```python
from build123d import *

# Parameters (mm, degrees)
SKETCH1_W           = 50
SKETCH1_H           = 80
BOSS_EXTRUDE1_DEPTH = 9.5
CUT_EXTRUDE1_DEPTH  = 10.5
CUT_EXTRUDE2_DEPTH  = 4


with BuildPart() as part:
    # Sketch1 → Boss-Extrude1 (new body)
    with BuildSketch(Plane(origin=(0, 0, 0), x_dir=(1, 0, 0), z_dir=(0, 1, 0))):
        Rectangle(SKETCH1_W, SKETCH1_H)
    extrude(amount=BOSS_EXTRUDE1_DEPTH)

    # Sketch2 → Cut-Extrude1 (cut, through all)
    with BuildSketch(Plane(origin=(0, 9.5, 0), x_dir=(1, 0, 0), z_dir=(0, 1, 0))):
        with BuildLine():
            Line((-13.9, 35), (-13.9, 31))
            ThreePointArc((-13.9, 31), (-15.5, 29.4), (-17.1, 31))
            Line((-17.1, 31), (-17.1, 35))
            ThreePointArc((-17.1, 35), (-15.5, 36.6), (-13.9, 35))
        make_face()
        with BuildLine():
            Line((13.9, 35), (13.9, 31))
            ThreePointArc((13.9, 31), (15.5, 29.4), (17.1, 31))
            Line((17.1, 31), (17.1, 35))
            ThreePointArc((17.1, 35), (15.5, 36.6), (13.9, 35))
        make_face()
        with BuildLine():
            Line((-13.9, 4), (-13.9, 0))
            ThreePointArc((-13.9, 0), (-15.5, -1.6), (-17.1, 0))
            Line((-17.1, 0), (-17.1, 4))
            ThreePointArc((-17.1, 4), (-15.5, 5.6), (-13.9, 4))
        make_face()
        with BuildLine():
            Line((13.9, 4), (13.9, 0))
            ThreePointArc((13.9, 0), (15.5, -1.6), (17.1, 0))
            Line((17.1, 0), (17.1, 4))
            ThreePointArc((17.1, 4), (15.5, 5.6), (13.9, 4))
        make_face()
        with BuildLine():
            Line((8.5, 19.5), (8.5, 15.5))
            ThreePointArc((8.5, 15.5), (0, 7), (-8.5, 15.5))
            Line((-8.5, 15.5), (-8.5, 19.5))
            ThreePointArc((-8.5, 19.5), (0, 28), (8.5, 19.5))
        make_face()
    extrude(amount=-CUT_EXTRUDE1_DEPTH, mode=Mode.SUBTRACT)

    # Sketch3 → Cut-Extrude2 (cut)
    with BuildSketch(Plane(origin=(0, 9.5, 0), x_dir=(1, 0, 0), z_dir=(0, 1, 0))):
        with BuildLine():
            Line((12, 19.5), (12, 15.358826141))
            ThreePointArc((12, 15.358826141), (0, 3.358826141), (-12, 15.358826141))
            Line((-12, 15.358826141), (-12, 19.5))
            ThreePointArc((-12, 19.5), (0, 31.5), (12, 19.5))
        make_face()
    extrude(amount=-CUT_EXTRUDE2_DEPTH, mode=Mode.SUBTRACT)


solid = part.part
```
Work out the finished part from the listing and answer in its coordinate system (mm). A direction names the side the tool comes from. Coordinates: 2 decimals unless noted, no trailing zeros. Loops run counter-clockwise (first coordinate to the right, second up) from the corner with the lowest first, then second, coordinate; pieces in that order, holes last.
1) Section B-B (y = 2.75) is taken. Give the vertices of the cut face in (x, z).
Results:
outline: (-25, -40) - (25, -40) - (25, 40) - (-25, 40) - close; hole (-17.1, -35) arc R1.6 ccw to (-13.9, -35) - (-13.9, -31) arc R1.6 ccw to (-17.1, -31) - close; hole (-17.1, -4) arc R1.6 ccw to (-13.9, -4) - (-13.9, 0) arc R1.6 ccw to (-17.1, 0) - close; hole (-8.5, -19.5) arc R8.5 ccw to (8.5, -19.5) - (8.5, -15.5) arc R8.5 ccw to (-8.5, -15.5) - close; hole (13.9, -35) arc R1.6 ccw to (17.1, -35) - (17.1, -31) arc R1.6 ccw to (13.9, -31) - close; hole (13.9, -4) arc R1.6 ccw to (17.1, -4) - (17.1, 0) arc R1.6 ccw to (13.9, 0) - close
2) Section A-A (x = 15.5) is taken. Give the vertices of the cut face in (y, z).
Results:
outline: (0, -40) - (9.5, -40) - (9.5, -36.6) - (0, -36.6) - close; (0, -29.4) - (9.5, -29.4) - (9.5, -5.6) - (0, -5.6) - close; (0, 1.6) - (9.5, 1.6) - (9.5, 40) - (0, 40) - close
3) For faces 4 (the cylindrical face through (-0.264, 7.528, -31.497)), 5 (the flat face through (-13.9, 5, -2)), determine the directions among +Z, -Z, +X, -X, +Y, -Y from which every point of the face is accessible in a straight line to the end or side of a thin tool.
Results:
face 4: +Y
face 5: +Y, -Y
4) Consider probe 1 along X at (y, z) = (6, -32); probe 2 along Z at (x, y) = (15.5, 8); probe 3 along Z at (x, y) = (-0.5, 5). Determine where each line is inside the solid, lowest interval first.
Results:
probe 1: x = -25 to -17.1, -13.9 to 13.9, 17.1 to 25
probe 2: z = -40 to -36.6, -29.4 to -5.6, 1.6 to 40
probe 3: z = -40 to -27.99, -7.01 to 40
5) Section D-D (y = 8.5) is taken. Give the vertices of the cut face in (x, z), plus the area to 3 significant figures.
Results:
outline: (-25, -40) - (25, -40) - (25, 40) - (-25, 40) - close; hole (-17.1, -35) arc R1.6 ccw to (-13.9, -35) - (-13.9, -31) arc R1.6 ccw to (-17.1, -31) - close; hole (-17.1, -4) arc R1.6 ccw to (-13.9, -4) - (-13.9, 0) arc R1.6 ccw to (-17.1, 0) - close; hole (-12, -19.5) arc R12 ccw to (12, -19.5) - (12, -15.36) arc R12 ccw to (-12, -15.36) - close; hole (13.9, -35) arc R1.6 ccw to (17.1, -35) - (17.1, -31) arc R1.6 ccw to (13.9, -31) - close; hole (13.9, -4) arc R1.6 ccw to (17.1, -4) - (17.1, 0) arc R1.6 ccw to (13.9, 0) - close
area: 3,360 mm2
6) Section C-C (z = -24.5) is taken. Give the vertices of the cut face in (x, y), plus the area to 3 significant figures.
Results:
outline: (-25, 0) - (-6.87, 0) - (-6.87, 5.5) - (-10.91, 5.5) - (-10.91, 9.5) - (-25, 9.5) - close; (6.87, 0) - (25, 0) - (25, 9.5) - (10.91, 9.5) - (10.91, 5.5) - (6.87, 5.5) - close
area: 312 mm2
7) For a pull along Z with two mould halves and no side action, classify faces 1 (the flat face through (12, 8, -17)), 2 (the flat face through (0, 5, 40)), 3 (the flat face through (0, 0, -1)) as +Z half, -Z half, draft (parallel to the pull), parting line (faces both ways), or undercut.
Results:
face 1: undercut
face 2: +Z half
face 3: draft
